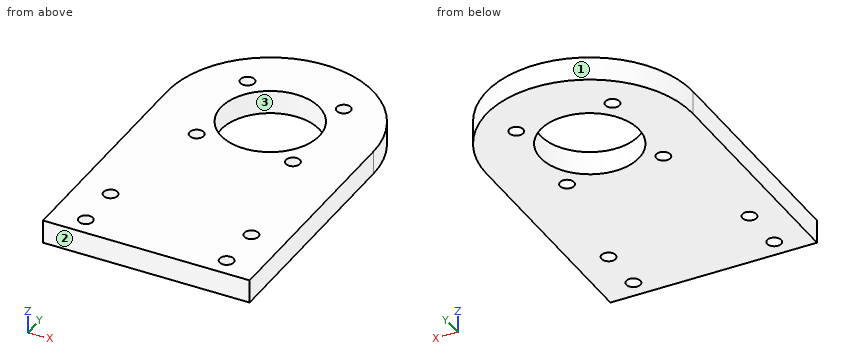
```python
from build123d import *

# Parameters (mm, degrees)
SKETCH_1_R          = 1.5
SKETCH_1_R_2        = 10.5
EXTRUDE_1_DEPTH     = 5
SKETCH_2_R          = 1.5
CUT_EXTRUDE_1_DEPTH = 6


with BuildPart() as part:
    # 草图1 → 凸台-拉伸1 (new body)
    with BuildSketch(Plane.XY):
        with BuildLine():
            Line((-22, 0), (22, 0))
            Line((22, 0), (22, 50))
            ThreePointArc((22, 50), (0, 72), (-22, 50))
            Line((-22, 50), (-22, 0))
        make_face()
        with Locations((-15, 14)):
            Circle(SKETCH_1_R, mode=Mode.SUBTRACT)
        with Locations((-15, 4)):
            Circle(SKETCH_1_R, mode=Mode.SUBTRACT)
        with Locations((15, 4)):
            Circle(SKETCH_1_R, mode=Mode.SUBTRACT)
        with Locations((15, 14)):
            Circle(SKETCH_1_R, mode=Mode.SUBTRACT)
        with Locations((0, 50)):
            Circle(SKETCH_1_R_2, mode=Mode.SUBTRACT)
    extrude(amount=EXTRUDE_1_DEPTH)

    # 草图2 → 切除-拉伸1 (cut, through all)
    with BuildSketch(Plane(origin=(0, 0, 0), x_dir=(-1, 0, 0), z_dir=(0, 0, -1))):
        with Locations((10.253048327, 60.253048327)):
            Circle(SKETCH_2_R)
        with Locations((10.253048327, 39.746951673)):
            Circle(SKETCH_2_R)
        with Locations((-10.253048327, 39.746951673)):
            Circle(SKETCH_2_R)
        with Locations((-10.253048327, 60.253048327)):
            Circle(SKETCH_2_R)
    extrude(amount=-CUT_EXTRUDE_1_DEPTH, mode=Mode.SUBTRACT)


solid = part.part
```
Source: CAD feature listing. Evaluate the final solid. Frame: model axes, mm. Face numbers are marked on the shaded views. Round coordinates to 2 decimals unless told otherwise and drop trailing zeros. Loops run counter-clockwise (first coordinate to the right, second up) from the corner with the lowest first, then second, coordinate; pieces in that order, holes last. Notation, with made-up numbers: M -32.75,-19 L -24.75,-19 A19 cw -24.75,12 Z; hole C -9,39 d8. An arc over 180 degrees is marked long. Put each result on its own line as item: value.
(1) Section D-D, the plane y = 55.5. Return loops of the section in (x, z).
Solutions:
outline: M -21.3,0 L -8.94,0 L -8.94,5 L -21.3,5 Z; M 8.94,0 L 21.3,0 L 21.3,5 L 8.94,5 Z
(2) Section A-A, the plane y = 4. Return loops of the section in (x, z).
Solutions:
outline: M -22,0 L -16.5,0 L -16.5,5 L -22,5 Z; M -13.5,0 L 13.5,0 L 13.5,5 L -13.5,5 Z; M 16.5,0 L 22,0 L 22,5 L 16.5,5 Z
(3) Pull-direction query (X, two-part tool) for the marked faces 1, 2 and 3; classes: released by +X, released by -X, zero draft, split by the parting line, or undercut.
Solutions:
face 1: split by the parting line
face 2: zero draft
face 3: undercut
(4) Section B-B, the plane x = -7. Return loops of the section in (y, z), and give its area (3 significant figures).
Solutions:
outline: M 0,0 L 42.17,0 L 42.17,5 L 0,5 Z; M 57.83,0 L 70.86,0 L 70.86,5 L 57.83,5 Z
area: 276 mm²
(5) Ray query, line 1 (Y direction, x = -11, z = 3.6); line 2 (Y direction, x = 16, z = 3.75); line 3 (Y direction, x = -9, z = 0.4). Return the intervals inside material, ascending. Write a range as [from, to].
Solutions:
line 1: [0, 38.45], [41.05, 58.95], [61.55, 69.05]
line 2: [0, 2.88], [5.12, 12.88], [15.12, 65.1]
line 3: [0, 38.92], [40.57, 44.59], [55.41, 59.43], [61.08, 70.07]
(6) First-contact query: pin 1 (2 mm diameter, centred on x = -3, z = 1.5, fed in from +Y); pin 2 (2 mm diameter, centred on x = 5, z = 1, fed in from +Y); pin 3 (1.5 mm diameter, centred on x = -4, z = 1.5, fed in from +Y). Flat tips, straight axial feed; report the tip coordinate or a pass-through.
Solutions:
pin 1: y = 71.91
pin 2: y = 71.63
pin 3: y = 71.76
(7) Section C-C, the plane z = 3.45. State how many separate pieces and enclosed holes the cut face has, and give its area (3 significant figures).
Solutions:
separate pieces: 1
enclosed holes: 9
area: 2,560 mm²
